Source: CAD feature listing. Evaluate the final solid. Frame: model axes, mm. Round coordinates to 2 decimals unless told otherwise and drop trailing zeros. Answer in a Markdown table with one row per item. Add a question column.
Item 1: Material intervals for probe 1 along Z at (x, y) = (118.5, 1.85); probe 2 along X at (y, z) = (2.5, 114.5), sorted ascending.
Item 2: Cut plane A-A on y = 2.45. Give the number of separate pieces and of enclosed holes in the cut face, and give its area (3 significant figures).
Item 3: Contact query for a flat-ended pin moving along its axis: pin 1 (1.5 mm diameter, centred on y = 1, z = 141.5, fed in from +X). Output: stop coordinate, or through.
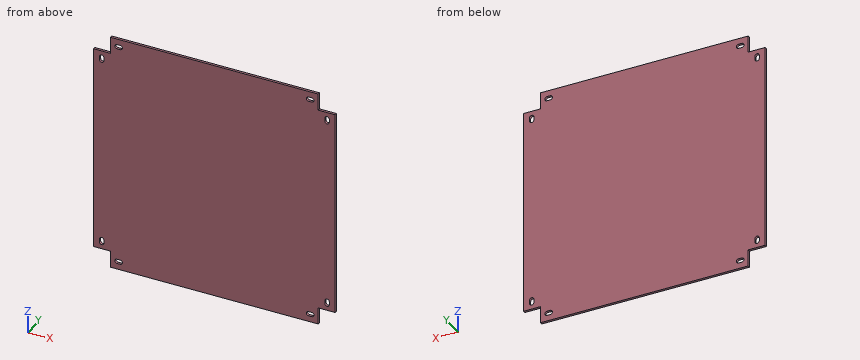
from build123d import *

# Parameters (mm, degrees)
BOSS_EXTRUDE1_DEPTH = 3


with BuildPart() as part:
    # Sketch1 → Boss-Extrude1 (new body)
    with BuildSketch(Plane(origin=(0, 0, 0), x_dir=(1, 0, 0), z_dir=(0, 1, 0))):
        Polygon((-129, -129), (-129, -150), (129, -150), (129, -129), (150, -129), (150, 129), (129, 129), (129, 150), (-129, 150), (-129, 129), (-150, 129), (-150, -129), align=None)
        with BuildLine():
            Line((-117, -142.75), (-121, -142.75))
            ThreePointArc((-121, -142.75), (-123.75, -140), (-121, -137.25))
            Line((-121, -137.25), (-117, -137.25))
            ThreePointArc((-117, -137.25), (-114.25, -140), (-117, -142.75))
        make_face(mode=Mode.SUBTRACT)
        with BuildLine():
            Line((-137.25, -117), (-137.25, -121))
            ThreePointArc((-137.25, -121), (-140, -123.75), (-142.75, -121))
            Line((-142.75, -121), (-142.75, -117))
            ThreePointArc((-142.75, -117), (-140, -114.25), (-137.25, -117))
        make_face(mode=Mode.SUBTRACT)
        with BuildLine():
            ThreePointArc((121, -137.25), (123.75, -140), (121, -142.75))
            Line((121, -142.75), (117, -142.75))
            ThreePointArc((117, -142.75), (114.25, -140), (117, -137.25))
            Line((117, -137.25), (121, -137.25))
        make_face(mode=Mode.SUBTRACT)
        with BuildLine():
            ThreePointArc((142.75, -121), (140, -123.75), (137.25, -121))
            Line((137.25, -121), (137.25, -117))
            ThreePointArc((137.25, -117), (140, -114.25), (142.75, -117))
            Line((142.75, -117), (142.75, -121))
        make_face(mode=Mode.SUBTRACT)
        with BuildLine():
            ThreePointArc((-142.75, 121), (-140, 123.75), (-137.25, 121))
            Line((-137.25, 121), (-137.25, 117))
            ThreePointArc((-137.25, 117), (-140, 114.25), (-142.75, 117))
            Line((-142.75, 117), (-142.75, 121))
        make_face(mode=Mode.SUBTRACT)
        with BuildLine():
            ThreePointArc((-121, 137.25), (-123.75, 140), (-121, 142.75))
            Line((-121, 142.75), (-117, 142.75))
            ThreePointArc((-117, 142.75), (-114.25, 140), (-117, 137.25))
            Line((-117, 137.25), (-121, 137.25))
        make_face(mode=Mode.SUBTRACT)
        with BuildLine():
            Line((137.25, 117), (137.25, 121))
            ThreePointArc((137.25, 121), (140, 123.75), (142.75, 121))
            Line((142.75, 121), (142.75, 117))
            ThreePointArc((142.75, 117), (140, 114.25), (137.25, 117))
        make_face(mode=Mode.SUBTRACT)
        with BuildLine():
            Line((117, 142.75), (121, 142.75))
            ThreePointArc((121, 142.75), (123.75, 140), (121, 137.25))
            Line((121, 137.25), (117, 137.25))
            ThreePointArc((117, 137.25), (114.25, 140), (117, 142.75))
        make_face(mode=Mode.SUBTRACT)
    extrude(amount=BOSS_EXTRUDE1_DEPTH)


solid = part.part
Results below:
| question | item | result |
|---|---|---|
| 1 | probe 1 | -150 to -142.75, -137.25 to 137.25, 142.75 to 150 |
| 1 | probe 2 | -150 to -141.15, -138.85 to 138.85, 141.15 to 150 |
| 2 | separate pieces | 1 |
| 2 | enclosed holes | 8 |
| 2 | area | 87,900 mm2 |
| 3 | pin 1 | x = 129 |
